The model under review builds one solid part; all positions refer to its coordinate system, in mm. Face numbers are marked on the shaded views. A direction names the side the tool comes from. Give positions to 0.01 mm unless a question says otherwise; leave off trailing zeros. Loops run counter-clockwise (first coordinate to the right, second up) from the corner with the lowest first, then second, coordinate; pieces in that order, holes last. Notation, with made-up numbers: (79.5, 50.25) - (124.5, 50.25) arc R26 ccw to (124.5, 86.25) - close; hole circle Ø7 at (30.5, 60.25). An arc over 180 degrees is marked (long way). Return JSON: item names as keys, results as strings. Group by question number.
```python
from build123d import *

# Parameters (mm, degrees)
F0_R     = 11
F0_R_2   = 4
F1_DEPTH = 3.5
F2_SIZE  = 1
F4_DEPTH = 7.001


# Not quite as in the source:
# - a feature names something its author has since deleted; it is built from what else it names


with BuildPart() as f1:
    # F0 (on Top) → F1 (new body, symmetric)
    with BuildSketch(Plane.XY):
        with BuildLine():
            ThreePointArc((-6, 11.5325625947), (0, 13), (6, 11.5325625947))
            Line((6, 11.5325625947), (6, 33))
            ThreePointArc((6, 33), (0, 27), (-6, 33))
            Line((-6, 33), (-6, 11.5325625947))
        make_face()
        with BuildLine():
            ThreePointArc((-6.9874921777, -10.96243372), (-11.2583302492, -6.5), (-12.9874921777, -0.5701288746))
            Line((-12.9874921777, -0.5701288746), (-31.5788383249, -11.3038475773))
            ThreePointArc((-31.5788383249, -11.3038475773), (-25.5788383249, -11.3038475773), (-22.5788383249, -16.5))
            ThreePointArc((-22.5788383249, -16.5), (-23.3826859022, -19.5), (-25.5788383249, -21.6961524227))
            Line((-25.5788383249, -21.6961524227), (-6.9874921777, -10.96243372))
        make_face()
        with BuildLine():
            Line((31.5788383249, -11.3038475773), (12.9874921777, -0.5701288746))
            ThreePointArc((12.9874921777, -0.5701288746), (11.2583302492, -6.5), (6.9874921777, -10.96243372))
            Line((6.9874921777, -10.96243372), (25.5788383249, -21.6961524227))
            ThreePointArc((25.5788383249, -21.6961524227), (23.3826859022, -13.5), (31.5788383249, -11.3038475773))
        make_face()
        with BuildLine():
            ThreePointArc((12.9874921777, -0.5701288746), (12.9968726683, -0.2851330301), (13, 0))
            ThreePointArc((13, 0), (11.1130553854, 6.7453687816), (6, 11.5325625947))
            ThreePointArc((6, 11.5325625947), (0, 13), (-6, 11.5325625947))
            ThreePointArc((-6, 11.5325625947), (-11.2583302492, 6.5), (-12.9874921777, -0.5701288746))
            ThreePointArc((-12.9874921777, -0.5701288746), (-11.2583302492, -6.5), (-6.9874921777, -10.96243372))
            ThreePointArc((-6.9874921777, -10.96243372), (0, -13), (6.9874921777, -10.96243372))
            ThreePointArc((6.9874921777, -10.96243372), (11.2583302492, -6.5), (12.9874921777, -0.5701288746))
        make_face()
        Circle(F0_R, mode=Mode.SUBTRACT)
        with BuildLine():
            ThreePointArc((-6, 33), (0, 27), (6, 33))
            ThreePointArc((6, 33), (0, 39), (-6, 33))
        make_face()
        with Locations((0, 33)):
            Circle(F0_R_2, mode=Mode.SUBTRACT)
        with BuildLine():
            ThreePointArc((-22.5788383249, -16.5), (-25.5788383249, -11.3038475773), (-31.5788383249, -11.3038475773))
            ThreePointArc((-31.5788383249, -11.3038475773), (-33.7749907476, -19.5), (-25.5788383249, -21.6961524227))
            ThreePointArc((-25.5788383249, -21.6961524227), (-23.3826859022, -19.5), (-22.5788383249, -16.5))
        make_face()
        with Locations((-28.5788383249, -16.5)):
            Circle(F0_R_2, mode=Mode.SUBTRACT)
        with BuildLine():
            ThreePointArc((34.5788383249, -16.5), (33.7749907476, -13.5), (31.5788383249, -11.3038475773))
            ThreePointArc((31.5788383249, -11.3038475773), (23.3826859022, -13.5), (25.5788383249, -21.6961524227))
            ThreePointArc((25.5788383249, -21.6961524227), (31.5788383249, -21.6961524227), (34.5788383249, -16.5))
        make_face()
        with Locations((28.5788383249, -16.5)):
            Circle(F0_R_2, mode=Mode.SUBTRACT)
    extrude(amount=F1_DEPTH, both=True)

    # F2
    f2_edges = [f1.edges().sort_by_distance(p)[0] for p in [
        (-4, 33, 3.5),
        (-11, 0, 3.5),
        (-32.578838, -16.5, 3.5),
        (24.578838, -16.5, 3.5),
        (-32.578838, -16.5, -3.5),
        (-11, 0, -3.5),
        (24.578838, -16.5, -3.5),
        (-4, 33, -3.5),
    ]]
    chamfer(f2_edges, length=F2_SIZE)

    # F3 (on face) → F4 (cut, through all)
    with BuildSketch(Plane.XY.offset(3.5)):
        with BuildLine():
            Line((4, 12.3693168769), (4, 28.527864045))
            ThreePointArc((4, 28.527864045), (0, 27), (-4, 28.527864045))
            Line((-4, 28.527864045), (-4, 12.3693168769))
            ThreePointArc((-4, 12.3693168769), (0, 13), (4, 12.3693168769))
        make_face()
        with BuildLine():
            ThreePointArc((-8.7121426428, -9.6487600536), (-11.2583302492, -6.5), (-12.7121426428, -2.7205568233))
            Line((-12.7121426428, -2.7205568233), (-26.7058549787, -10.7998304074))
            ThreePointArc((-26.7058549787, -10.7998304074), (-23.7189051938, -12.9813283811), (-22.5788383249, -16.5))
            ThreePointArc((-22.5788383249, -16.5), (-22.6106769632, -17.117292444), (-22.7058549787, -17.7280336376))
            Line((-22.7058549787, -17.7280336376), (-8.7121426428, -9.6487600536))
        make_face()
        with BuildLine():
            Line((26.7058549787, -10.7998304074), (12.7121426428, -2.7205568233))
            ThreePointArc((12.7121426428, -2.7205568233), (11.2583302492, -6.5), (8.7121426428, -9.6487600536))
            Line((8.7121426428, -9.6487600536), (22.7058549787, -17.7280336376))
            ThreePointArc((22.7058549787, -17.7280336376), (23.3826859022, -13.5), (26.7058549787, -10.7998304074))
        make_face()
    extrude(amount=-F4_DEPTH, mode=Mode.SUBTRACT)


solid = f1.part
```
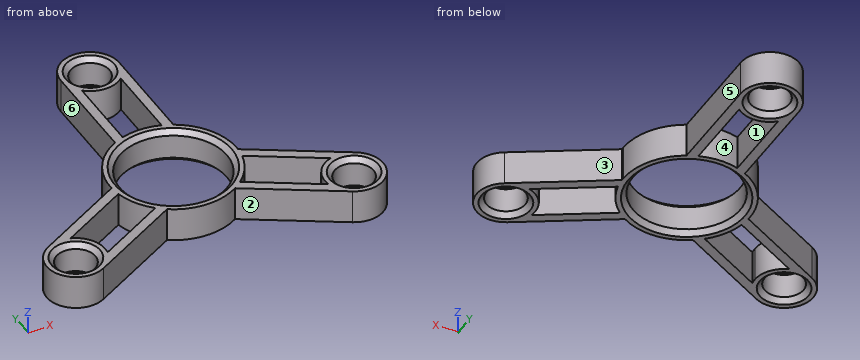
1) We need section C-C, the plane z = -0.75. Write out the cut boundary in (x, y), plus the area to 3 significant figures.
2) For pin 1 Ø2 at (y, z) = (23.5, 1.5) entering from +X; pin 2 Ø1 at (y, z) = (8, -1.5) entering from -X; pin 3 Ø2 at (y, z) = (8.5, -2) entering from +X, all flat-tipped, find the tip position at first contact; note any pin that passes through.
3) We need section B-B, the plane x = 0. Write out the cut boundary in (y, z), plus the area to 3 significant figures.
4) Tool access review of the marked faces 1, 2 and 3: name each direction out of +Z, -Z, +X, -X, +Y, -Y from which nothing blocks a thin tool from reaching the whole face with its end or side.
5) Draft analysis for pull direction X (two halves, no side actions). For the marked faces 4, 5 and 6, state which applies: +X half, -X half, draft (parallel to the pull), parting line (faces both ways), or undercut.
6) To check wall thickness, follow line 1 (Y direction, x = 25, z = -0.5); line 2 (X direction, y = -8, z = 3.25); line 3 (Y direction, x = -26, z = -2.25). State the ranges of each line that lie inside material, in increasing order.
7) We need section A-A, the plane y = 22.5. Write out the cut boundary in (x, z).
8) We need section D-D, the plane y = -7.5. Count the separate pieces of the cut face and the enclosed holes in it, plus the area to 3 significant figures.
Findings:
{
 "1": {"outline": "(-31.58, -11.3) arc R6 ccw to (-25.58, -21.7) - (-6.99, -10.96) arc R13 ccw to (6.99, -10.96) - (25.58, -21.7) arc R6 ccw to (31.58, -11.3) - (12.99, -0.57) arc R13 ccw to (6, 11.53) - (6, 33) arc R6 ccw to (-6, 33) - (-6, 11.53) arc R13 ccw to (-12.99, -0.57) - close; hole circle Ø8 at (-28.58, -16.5); hole (-26.71, -10.8) arc R6 cw to (-22.71, -17.73) - (-8.71, -9.65) arc R13 cw to (-12.71, -2.72) - close; hole circle Ø22 at (0, 0); hole (-4, 12.37) arc R13 cw to (4, 12.37) - (4, 28.53) arc R6 cw to (-4, 28.53) - close; hole circle Ø8 at (0, 33); hole (8.71, -9.65) - (22.71, -17.73) arc R6 cw to (26.71, -10.8) - (12.71, -2.72) arc R13 cw to start; hole circle Ø8 at (28.58, -16.5)", "area": "554 mm^2"},
 "2": {"pin 1": "stops at x = 6", "pin 2": "stops at x = -10.62", "pin 3": "stops at x = 10.62"},
 "3": {"outline": "(-13, -3.5) - (-12, -3.5) - (-11, -2.5) - (-11, 2.5) - (-12, 3.5) - (-13, 3.5) - close; (11, -2.5) - (12, -3.5) - (13, -3.5) - (13, 3.5) - (12, 3.5) - (11, 2.5) - close; (27, -3.5) - (28, -3.5) - (29, -2.5) - (29, 2.5) - (28, 3.5) - (27, 3.5) - close; (37, -2.5) - (38, -3.5) - (39, -3.5) - (39, 3.5) - (38, 3.5) - (37, 2.5) - close", "area": "52.0 mm^2"},
 "4": {"face 1": "+Z, -Z", "face 2": "+Z, -Z, -Y", "face 3": "+Z, -Z, +X, +Y"},
 "5": {"face 4": "undercut", "face 5": "+X half", "face 6": "-X half"},
 "6": {"line 1": "y = -21.36 to -18.29, -14.71 to -11.68, -9.81 to -7.51", "line 2": "x = -25.86 to -21.86, -10.25 to -8.61, 8.61 to 10.25, 21.86 to 25.86", "line 3": "y = -21.92 to -19.56, -13.44 to -11.08, -10.39 to -8.08"},
 "7": {"outline": "(-6, -3.5) - (-4, -3.5) - (-4, 3.5) - (-6, 3.5) - close; (4, -3.5) - (6, -3.5) - (6, 3.5) - (4, 3.5) - close"},
 "8": {"separate pieces": "4", "enclosed holes": "0", "area": "89.3 mm^2"}
}
